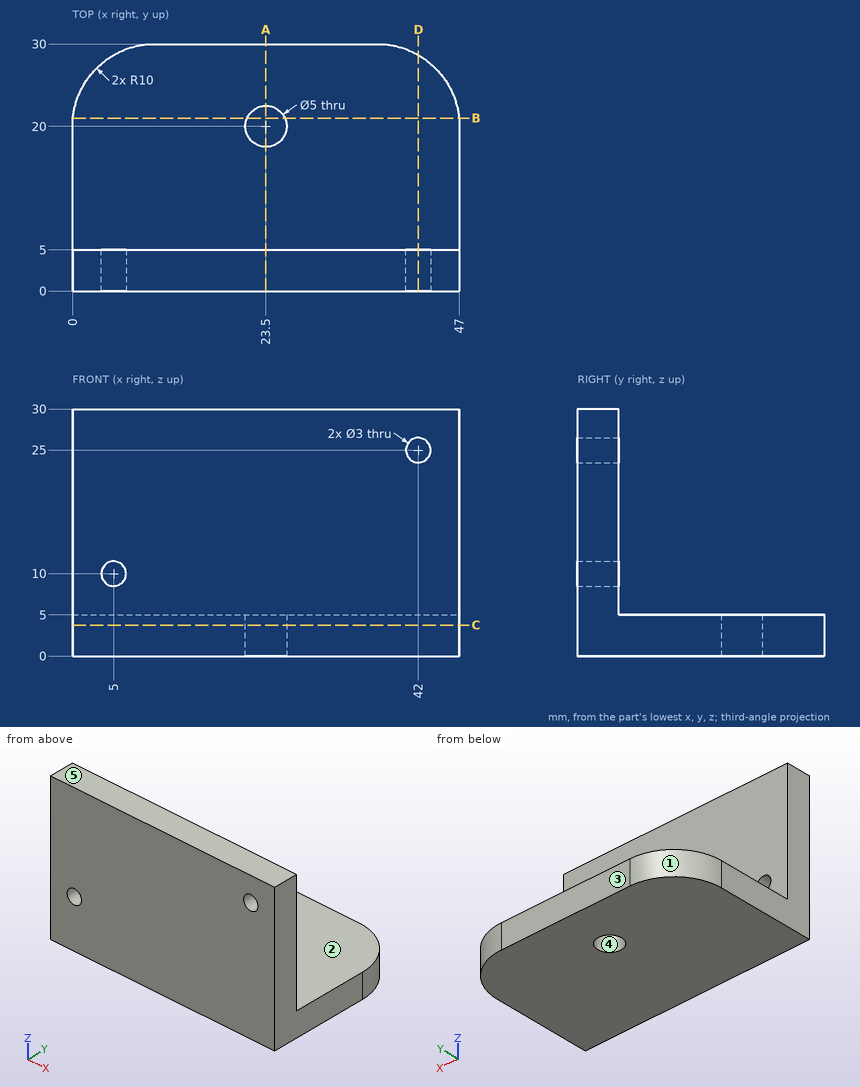
Can you work these out from the drawing? Everything is in mm from the part's minimum corner. A direction names the side the tool comes from. Give positions to 0.01 mm unless a question says otherwise; leave off trailing zeros. Order: outer loops, then holes, each group sorted by start corner. A loop starts at its lowest first (then second) coordinate and runs counter-clockwise, first axis right, second up.
Item 1: If we mould it in two halves opening along Y, with no side actions, what happens to the marked faces 3, 4 and 5? For each: pulls with the +Y half, pulls with the -Y half, needs draft (parallel to the pull), parting line crosses it, or undercut.
Item 2: If we section it at D-D, the plane x = 42: Write out the boundary of the cut face in (y, z).
Item 3: For the marked faces 1 and 2, which set-ups out of +Z, -Z, +X, -X, +Y, -Y let a thin tool reach every point of the face, with its end or its side?
Item 4: If we section it at A-A, the plane x = 23.5: Write out the boundary of the cut face in (y, z), plus the area to 3 significant figures.
Item 5: I need wall thicknesses on line 1 (Y direction, x = 23.5, z = 4); line 2 (X direction, y = 20, z = 3.65); line 3 (Z direction, x = 42, y = 2). Which ranges of each line are inside material? Lowest first, please.
Item 6: If we section it at B-B, the plane y = 21: Write out the boundary of the cut face in (x, z), plus the area to 3 significant figures.
Item 7: If we section it at C-C, the plane z = 3.75: Write out the boundary of the cut face in (x, y).
Item 8: I'm going to push flat-ended pins straight in: pin 1 (12.5 mm diameter, centred on x = 30.5, y = 12, fed in from +Z); pin 2 (6 mm diameter, centred on x = 34.5, z = 19, fed in from +Y). Where does each tip first touch, or does it pass through?
Values:
1. face 3: pulls with the +Y half
1. face 4: undercut
1. face 5: needs draft
2. outline: (0, 0) - (28.66, 0) - (28.66, 5) - (5, 5) - (5, 23.5) - (0, 23.5) - close; (0, 26.5) - (5, 26.5) - (5, 30) - (0, 30) - close
3. face 1: +Z, -Z, -X, +Y
3. face 2: +Z, +X, -X, +Y
4. outline: (0, 0) - (17.5, 0) - (17.5, 5) - (5, 5) - (5, 30) - (0, 30) - close; (22.5, 0) - (30, 0) - (30, 5) - (22.5, 5) - close
4. area: 250 mm2
5. line 1: y = 0 to 17.5, 22.5 to 30
5. line 2: x = 0 to 21, 26 to 47
5. line 3: z = 0 to 23.5, 26.5 to 30
6. outline: (0.05, 0) - (21.21, 0) - (21.21, 5) - (0.05, 5) - close; (25.79, 0) - (46.95, 0) - (46.95, 5) - (25.79, 5) - close
6. area: 212 mm2
7. outline: (0, 0) - (47, 0) - (47, 20) arc R10 ccw to (37, 30) - (10, 30) arc R10 ccw to (0, 20) - close; hole circle Ø5 at (23.5, 20)
8. pin 1: stops at z = 5
8. pin 2: stops at y = 5
